For this review, take the finished solid that the model builds, in its own axes (mm). A direction names the side the tool comes from. Round coordinates to 2 decimals unless told otherwise and drop trailing zeros. Order: outer loops, then holes, each group sorted by start corner. A loop starts at its lowest first (then second) coordinate and runs counter-clockwise, first axis right, second up. Notation, with made-up numbers: (30, 69.5) - (73, 69.5) arc R22 cw to (73, 75.5) - close; hole circle Ø9 at (-17.5, 73). An arc over 180 degrees is marked (long way). Write each question's results on one line, items separated by ' | '. Start each with the question number.
(1) Insertion check: pin 1 Ø6 at (y, z) = (1.5, 30.5) entering from -X; pin 2 Ø6 at (x, z) = (5.5, 96) entering from -Y; pin 3 Ø1.5 at (x, z) = (3, 68.5) entering from -Y; pin 4 Ø5 at (x, y) = (1.5, 1) entering from +Z. Each pin has a flat end and moves straight along its axis. Give the tip position at first contact, or say it passes through.
(2) Take a section at A-A, the plane z = 55. Give the boundary of the cut face in (x, y), plus the area to 3 significant figures.
(3) For L1, parallel to Y at x = 0, z = 53.5; L2, parallel to Z at x = 3.25, y = 5.5; L3, parallel to Z at x = -3, y = 3.25, list the stretches that pass through material, from the lowest coordinate up. Write a range as from..to.
(4) For faces 1 (the flat face through (4, -4, 4)), 2 (the cylindrical face through (4.57, 7.167, 1.972)), list the 3-axis set-ups (+Z, -Z, +X, -X, +Y, -Y) from which the entire face can be reached by the end or side of a thin tool; tool diameter is ignored.
```python
from build123d import *

# Parameters (mm, degrees)
F0_R     = 8.5
F1_DEPTH = 4
F2_R     = 5
F3_DEPTH = 100
F8_R     = 0.5
F9_DEPTH = 112.7


with BuildPart() as f1:
    # F0 (on Top) → F1 (new body)
    with BuildSketch(Plane.XY):
        Circle(F0_R)
    extrude(amount=F1_DEPTH)

    # F2 (on Top) → F3 (join)
    with BuildSketch(Plane.XY):
        Circle(F2_R)
    extrude(amount=F3_DEPTH)

    # F4 (on Right) → F5 (revolve)
    with BuildSketch(Plane.YZ):
        Polygon((3, 105), (0, 105), (0, 100), (4, 100), align=None)
    revolve(axis=Axis((0, 0, 102.5), (0, 0, -1)))

    # F6 (on Right) → F7 (revolve)
    with BuildSketch(Plane.YZ):
        with BuildLine():
            Line((1, 107), (0, 107))
            Line((0, 107), (0, 105))
            Line((0, 105), (3, 105))
            ThreePointArc((3, 105), (2.414214, 106.414214), (1, 107))
        make_face()
    revolve(axis=Axis((0, 0, 106), (0, 0, -1)))

    # F8 (on face) → F9 (cut)
    with BuildSketch(Plane.XY.offset(107)):
        Circle(F8_R)
    extrude(amount=-F9_DEPTH, mode=Mode.SUBTRACT)


solid = f1.part
```
Results below:
1) pin 1: stops at x = -5 | pin 2: stops at y = -4.33 | pin 3: stops at y = -4.47 | pin 4: stops at z = 107
2) outline: circle Ø10 at (0, 0); hole circle Ø1 at (0, 0) | area: 77.8 mm^2
3) L1: y = -5..-0.5, 0.5..5 | L2: z = 0..4 | L3: z = 0..100
4) face 1: +Z | face 2: +Z, -Z
